Design review of the part built by this model. Coordinates are the model's own, in mm. A direction names the side the tool comes from. Give positions to 0.01 mm unless a question says otherwise; leave off trailing zeros. Order: outer loops, then holes, each group sorted by start corner. A loop starts at its lowest first (then second) coordinate and runs counter-clockwise, first axis right, second up. Notation, with made-up numbers: (19.5, 2.5) -> (61.5, 2.5) arc R12 cw to (61.5, 17.5) -> close; hole circle Ø4 at (-18, -26.5). An arc over 180 degrees is marked (long way). Return JSON: item names as keys, results as strings.
```python
from build123d import *

# Parameters (mm, degrees)
SKETCH1_R           = 3.5
SKETCH1_R_2         = 2.5
BOSS_EXTRUDE1_DEPTH = 10
SKETCH2_R           = 2.5
BOSS_EXTRUDE2_DEPTH = 3.75
SKETCH3_R           = 2.5
BOSS_EXTRUDE3_DEPTH = 200


with BuildPart() as part:
    # Sketch1 → Boss-Extrude1 (new body)
    with BuildSketch(Plane(origin=(0, 0, 0), x_dir=(1, 0, 0), z_dir=(0, 1, 0))):
        with Locations(Location((0, 0, 0), (0, 0, 270))):
            Circle(SKETCH1_R)
        with Locations(Location((0, 0, 0), (0, 0, 270))):
            Circle(SKETCH1_R_2, mode=Mode.SUBTRACT)
    extrude(amount=BOSS_EXTRUDE1_DEPTH)

    # Sketch2 → Boss-Extrude2 (add, symmetric)
    with BuildSketch(Plane(origin=(0, 10, 0), x_dir=(1, 0, 0), z_dir=(0, 1, 0))):
        with Locations(Location((0, 0, 0), (0, 0, 270))):
            Circle(SKETCH2_R)
    extrude(amount=BOSS_EXTRUDE2_DEPTH, both=True)

    # Sketch3 → Boss-Extrude3 (add)
    with BuildSketch(Plane(origin=(0, 13.75, 0), x_dir=(1, 0, 0), z_dir=(0, 1, 0))):
        with Locations(Location((0, 0, 0), (0, 0, 270))):
            Circle(SKETCH3_R)
    extrude(amount=BOSS_EXTRUDE3_DEPTH)


solid = part.part
```
Item 1: Mouldability with a two-part tool opening along X and no side actions: class faces 4 (the face through (-3.417, 4.93, -0.759)), 5 (the face through (0, 6.25, 0)), 6 (the face through (0, 213.75, 0)) as released by +X, released by -X, zero draft, split by the parting line, or undercut.
Result set:
{"face 4": "split by the parting line", "face 5": "undercut", "face 6": "zero draft"}
Item 2: Add section B-B (z = 0). Give the boundary of the cut face in (x, y), plus the area to 3 significant figures.
Result set:
{"outline": "(-3.5, 0) -> (-2.5, 0) -> (-2.5, 6.25) -> (2.5, 6.25) -> (2.5, 0) -> (3.5, 0) -> (3.5, 10) -> (2.5, 10) -> (2.5, 213.75) -> (-2.5, 213.75) -> (-2.5, 10) -> (-3.5, 10) -> close", "area": "1,060 mm^2"}
Item 3: For pin 1 (2 mm diameter, centred on y = 72, z = 0.5, fed in from +X); pin 2 (1.5 mm diameter, centred on x = 1, y = 76.5, fed in from +Z), all flat-tipped, find the tip position at first contact; note any pin that passes through.
Result set:
{"pin 1": "stops at x = 2.5", "pin 2": "stops at z = 2.49"}
Item 4: Add section A-A (x = 0). Give the boundary of the cut face in (y, z), plus the area to 3 significant figures.
Result set:
{"outline": "(0, -3.5) -> (10, -3.5) -> (10, -2.5) -> (213.75, -2.5) -> (213.75, 2.5) -> (10, 2.5) -> (10, 3.5) -> (0, 3.5) -> (0, 2.5) -> (6.25, 2.5) -> (6.25, -2.5) -> (0, -2.5) -> close", "area": "1,060 mm^2"}
Item 5: Machinability: for faces 1 (the face through (-2, 0, 2)), 2 (the face through (-2, 10, 2)), 3 (the face through (-2.44, 3.08, -0.54)), which of the approach directions +Z, -Z, +X, -X, +Y, -Y give a long, thin tool a straight path to every point of the face, cutting with its end or side? Answer none if there is none.
Result set:
{"face 1": "+Z, -Z, +X, -X, -Y", "face 2": "+Y", "face 3": "-Y"}
Item 6: Wall thickness on L1, parallel to X at y = 4.25, z = 0; L2, parallel to Y at x = -1.5, z = 1.5; L3, parallel to Y at x = -1, z = -2.5: over which ranges is each line inside the solid? List them lowest first. Write a range as [from, to].
Result set:
{"L1": "x = [-3.5, -2.5], [2.5, 3.5]", "L2": "y = [6.25, 213.75]", "L3": "y = [0, 10]"}
Item 7: Add section C-C (y = 115). Give the boundary of the cut face in (x, z), plus the area to 3 significant figures.
Result set:
{"outline": "circle Ø5 at (0, 0)", "area": "19.6 mm^2"}
